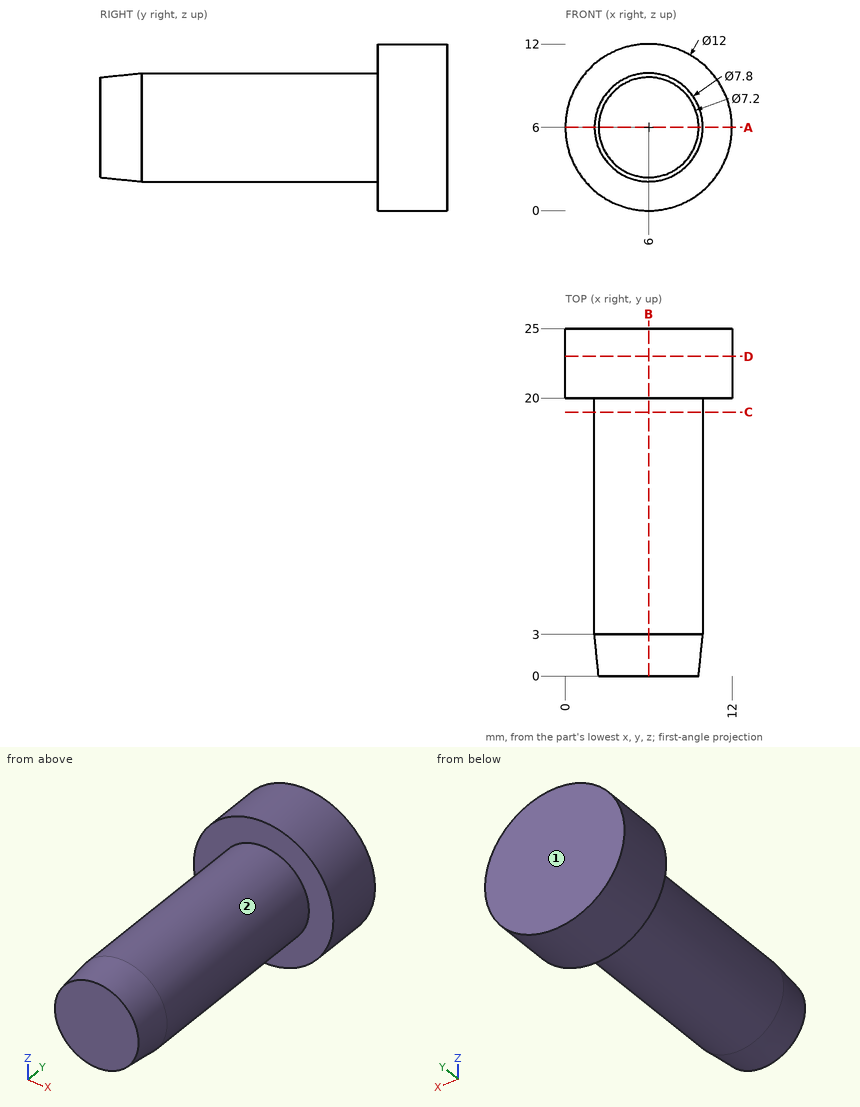
Geometry check sheet. Reference: drawing and pictorial views, mm from the part's lowest x, y, z. A direction names the side the tool comes from. Coordinates: 2 decimals unless noted, no trailing zeros. Write each loop counter-clockwise with the first axis right and the second up, starting at its lowest first coordinate (ties: lowest second). Pieces come first, ordered by that corner, then holes. Notation, with made-up numbers: (0, -16.75) -> (21, -16.75) arc R10 cw to (21, -8.75) -> close; hole circle Ø10 at (29, -20). An arc over 180 degrees is marked (long way). Use a Markdown table: item, result.
1. Sectioned sample at A-A (z = 6). Enter the section's corners in (x, y), plus the area to 3 significant figures.
Reported:
| item | result |
|---|---|
| outline | (0, 20) -> (2.1, 20) -> (2.1, 3) -> (2.4, 0) -> (9.6, 0) -> (9.9, 3) -> (9.9, 20) -> (12, 20) -> (12, 25) -> (0, 25) -> close |
| area | 215 mm2 |
2. Scan lines: line 1 along Y through (x, z) = (1.5, 8); line 2 along X through (y, z) = (13.25, 4.5). Record each from-to range of solid material in increasing order.
Reported:
| item | result |
|---|---|
| line 1 | y = 20 to 25 |
| line 2 | x = 2.4 to 9.6 |
3. Tool access check on the marked faces 1 and 2. Record the directions out of +Z, -Z, +X, -X, +Y, -Y that give a thin tool (end or side, any length) a straight path to the whole face; none if there is none.
Reported:
| item | result |
|---|---|
| face 1 | +Z, -Z, +X, -X, +Y |
| face 2 | -Y |
4. Sectioned sample at D-D (y = 23). Enter the section's corners in (x, z), plus the area to 3 significant figures.
Reported:
| item | result |
|---|---|
| outline | circle Ø12 at (6, 6) |
| area | 113 mm2 |
5. Sectioned sample at C-C (y = 19). Enter the section's corners in (x, z), plus the area to 3 significant figures.
Reported:
| item | result |
|---|---|
| outline | circle Ø7.8 at (6, 6) |
| area | 47.8 mm2 |
6. Sectioned sample at B-B (x = 6). Enter the section's corners in (y, z).
Reported:
| item | result |
|---|---|
| outline | (0, 2.4) -> (3, 2.1) -> (20, 2.1) -> (20, 0) -> (25, 0) -> (25, 12) -> (20, 12) -> (20, 9.9) -> (3, 9.9) -> (0, 9.6) -> close |
7. Go/stop test with flat-tipped pins: pin 1 Ø6 at (x, y) = (8, 16) entering from -Z; pin 2 Ø6 at (x, z) = (3, 7) entering from -Y; pin 3 Ø5 at (x, y) = (3, 2.5) entering from +Z. Record where each tip stops, or that it passes through.
Reported:
| item | result |
|---|---|
| pin 1 | stops at z = 2.1 |
| pin 2 | stops at y = 0 |
| pin 3 | stops at z = 9.86 |
